Read the model definition and answer for the solid it produces. Units are mm, in the model's axes. A direction names the side the tool comes from. Give positions to 0.01 mm unless a question says otherwise; leave off trailing zeros. Write each loop counter-clockwise with the first axis right and the second up, starting at its lowest first coordinate (ties: lowest second). Pieces come first, ordered by that corner, then holes.
Autodesk Inventor part; units mm, degrees
ref_plane "YZ Plane" through (0, 0, 0) normal (1, 0, 0) x (0, 1, 0)
ref_plane "XZ Plane" through (0, 0, 0) normal (0, 1, 0) x (-1, 0, 0)
ref_plane "XY Plane" through (0, 0, 0) normal (0, 0, 1) x (1, 0, 0)
sketch "Sketch1" plane through (0, 0, 0) normal (0, 0, 1) x (1, 0, 0)
  line L0 (-490, 48) -> (490, 48)
  line L1 (490, 48) -> (490, 0)
  line L2 (490, 0) -> (-490, 0)
  line L3 (-490, 0) -> (-490, 48)
  point P0 (0, 0)
  point P1 (0, 0)
  dimension "d0" = 980
  dimension "d1" = 48
extrude "Plate1" add sketch "Sketch1" along normal blind 2
sketch "Sketch2" plane through (490, -2, 0) normal (0, 1, 0) x (-1, 0, 0)
  line L0 (980, 0) -> (0, 0)
  line L1 (0, 0) -> (0, 20)
  line L2 (0, 20) -> (980, 20)
  line L3 (980, 20) -> (980, 0)
edge flange "Flange1" height 20 angle 90 thickness 2 bend radius 2.75 thickness toward (0, 1, 0) relief round relief width 2 relief depth 1 edges at (0, 0, 2) wall of the first edge with corners at (-490, -2, 0) (490, -2, 0) (490, -2, 20) (-490, -2, 20)
bend "Bend1"
corner "Corner1"
sketch "Sketch5" plane through (0, 0, 0) normal (0, 0, -1) x (-1, 0, 0)
  line L0 (490, 48) -> (-490, 48)
  line L1 (490, -2) -> (-490, -2)
  circle A0 centre (0, 48) radius 17.5
  line L2 (243.4, 48) -> (246.6, 48)
  line L3 (246.6, 48) -> (246.6, 26)
  line L4 (246.6, 26) -> (243.4, 26)
  line L5 (243.4, 26) -> (243.4, 48)
  line L6 (-243.4, 48) -> (-246.6, 48)
  line L7 (-246.6, 48) -> (-246.6, 26)
  line L8 (-246.6, 26) -> (-243.4, 26)
  line L9 (-243.4, 26) -> (-243.4, 48)
  line L10 (0, 48) -> (0, -2) construction
  line L11 (490, -2) -> (490, 48)
  line L12 (-490, -2) -> (-490, 48)
  circle A1 centre (-490, 48) radius 17.5
  circle A2 centre (490, 48) radius 17.5
  point P0 (0, 0)
  point P1 (245, 26)
  point P2 (-245, 26)
  point P3 (246.6, 48)
  point P4 (-17.5, 48)
  point P5 (17.5, 48)
  point P6 (-246.6, 48)
  point P7 (472.5, 48)
  point P8 (490, 30.5)
  point P9 (-490, 30.5)
  point P10 (-472.5, 48)
  dimension "d45" = 35
  dimension "d48" = 3.2
  dimension "d49" = 490
  dimension "d51" = 28
  dimension "d52" = 22
extrude "Extrusion1" cut sketch "Sketch5" against normal through all contours L3 L4 L5 L0 | L0 L11 A2 | L9 L8 L7 L0 | L12 L0 A1 picked at (488.702, 36.4796) picked at (-478.4796, 46.702)
sketch "Sketch9" plane through (0, 0, 2) normal (0, 0, 1) x (1, 0, 0)
  line L0 (448.2795, 24.3045) -> (448.2795, 12.3045) construction
  line L1 (448.2795, 12.3045) -> (248.2795, 12.3045) construction
  line L2 (248.2795, 12.3045) -> (248.2795, 24.3045) construction
  line L3 (248.2795, 24.3045) -> (448.2795, 24.3045) construction
  line L4 (-490, 48) -> (490, 48)
  point P0 (0, 0)
  point P1 (1.05, 68)
  point P2 (490, 48)
  point P3 (-490, 48)
  dimension "d40" = 200
  dimension "d41" = 12
mark "Mark2"
equation "\"d2\" = Thickness"
equation "\"d3\" = BendReliefWidth"
equation "\"d4\" = BendReliefDepth"
equation "\"d5\" = MinimumRemnant"
equation "\"d6\" = TransitionRadius"
equation "\"d9\" = BendRadius"
equation "\"d10\" = CornerReliefSize"
equation "\"d11\" = GapSize"
equation "\"d12\" = JacobiRadiusSize"
equation "\"BendReliefWidth\" = Thickness"
equation "\"BendReliefDepth\" = 0.5 * Thickness"
equation "\"CornerReliefSize\" = 4 * Thickness"
equation "\"MinimumRemnant\" = 2 * Thickness"
equation "\"TransitionRadius\" = BendRadius"
equation "\"JacobiRadiusSize\" = BendRadius"
equation "\"GapSize\" = Thickness"
properties part number "MSC 342 stringer BOARD  ##" material "Stainless Steel"
Item 1: Section A-A (y = 38.5) is taken. Write down the section's boundary in (x, z), and give its area (3 significant figures).
Result set:
outline: (-475.3, 0) - (-246.6, 0) - (-246.6, 2) - (-475.3, 2) - close; (-243.4, 0) - (243.4, 0) - (243.4, 2) - (-243.4, 2) - close; (246.6, 0) - (475.3, 0) - (475.3, 2) - (246.6, 2) - close
area: 1,890 mm2
Item 2: Which of the six approach directions +Z, -Z, +X, -X, +Y, -Y give full straight-line access (tool end or side, diameter ignored) to faces 1 (the flat face through (490, 8, 1)), 2 (the flat face through (-7, 26, 2))?
Result set:
face 1: +Z, -Z, +X, +Y, -Y
face 2: +Z, +X, -X, +Y
Item 3: Section C-C (z = 14.75) is taken. Write down the section's boundary in (x, y), and give its area (3 significant figures).
Result set:
outline: (-490, -2) - (490, -2) - (490, 0) - (-490, 0) - close
area: 1,960 mm2
Item 4: Section B-B (x = 228) is taken. Write down the section's boundary in (y, z), and give its area (3 significant figures).
Result set:
outline: (-2, 4.75) arc R4.75 ccw to (2.75, 0) - (48, 0) - (48, 2) - (2.75, 2) arc R2.75 cw to (0, 4.75) - (0, 20) - (-2, 20) - close
area: 133 mm2
Item 5: Each of these flat-tipped pins is pushed along its axis until it touches: pin 1 Ø0.6 at (y, z) = (41.5, 1) entering from -X; pin 2 Ø3 at (x, y) = (-3.5, 13) entering from +Z; pin 3 Ø4 at (x, z) = (-382, 6) entering from +Y; pin 4 Ø4 at (x, z) = (123.5, 3.5) entering from +Y. Where does it stop, or does it pass through?
Result set:
pin 1: stops at x = -473.88
pin 2: stops at z = 2
pin 3: stops at y = 0.1
pin 4: stops at y = 48
Item 6: Find the intervals of material crossed by line 1 along Y through (x, z) = (-319, 11); line 2 along Z through (x, y) = (-79, 17.5); line 3 along Y through (x, z) = (162.5, 2.75), in increasing order.
Result set:
line 1: y = -2 to 0
line 2: z = 0 to 2
line 3: y = -1.56 to 0.86
